from build123d import *
from build123d.topology import SkipClean

# Parameters (mm, degrees)
SKETCH1_R                = 6
BOSS_EXTRUDE1_DEPTH      = 11
SKETCH2_R                = 6
BOSS_EXTRUDE2_DEPTH      = 8
CUT_EXTRUDE1_DEPTH       = 10
CUT_EXTRUDE1_DEPTH_BACK  = 3
SKETCH3_R                = 6
SKETCH3_R_2              = 3
SKETCH5_W                = 8.868099488
SKETCH5_H                = 25.092164851
CUT_EXTRUDE3_DEPTH       = 20.723082923
CUT_EXTRUDE2_START       = -3.3
CUT_EXTRUDE2_DEPTH       = 3.3
CUT_EXTRUDE5_DEPTH       = 2.5
BOSS_EXTRUDE3_REACH      = 18.961
BOSS_EXTRUDE3_END_RADIUS = 6
BOSS_EXTRUDE4_START      = -2.211146
BOSS_EXTRUDE4_DEPTH      = 2.211146
SKETCH10_R               = 3
CUT_EXTRUDE6_DEPTH       = 19.364367672
SKETCH12_R               = 4
SKETCH12_R_2             = 3
BOSS_EXTRUDE5_DEPTH      = 0.3
BOSS_EXTRUDE6_START      = -5
BOSS_EXTRUDE6_DEPTH      = 10
CUT_EXTRUDE12_DEPTH      = 19.364367672
CUT_EXTRUDE9_DEPTH       = 14.244940814
SKETCH15_OUTSIDE_W       = 23.236
SKETCH15_OUTSIDE_H       = 20.984
SKETCH15_OUTSIDE_W_2     = 17.302035992
SKETCH15_OUTSIDE_H_2     = 16.797371099
CUT_EXTRUDE10_DEPTH      = 19.748333259
SKETCH16_R               = 1
CUT_EXTRUDE11_DEPTH      = 19.748333259


with BuildPart() as part:
    # Sketch1 → Boss-Extrude1 (new body)
    with BuildSketch(Plane.XY):
        Circle(SKETCH1_R)
    extrude(amount=BOSS_EXTRUDE1_DEPTH)

    # Sketch2 → Boss-Extrude2 (add, symmetric)
    with BuildSketch(Plane(origin=(0, 0, 0), x_dir=(0, 0, -1), z_dir=(1, 0, 0))):
        Circle(SKETCH2_R)
    extrude(amount=BOSS_EXTRUDE2_DEPTH, both=True)

    # Sketch3 → Cut-Extrude1 (cut, two sides: drawn at the far end of the back side and taken through both)
    with BuildSketch(Plane.ZY.offset(8).offset(-CUT_EXTRUDE1_DEPTH_BACK)):
        with Locations(Location((0, 0, 0), (0, 0, 33.557309762))):
            Circle(SKETCH3_R)
        with Locations(Location((0, 0, 0), (0, 0, 180))):
            Circle(SKETCH3_R_2, mode=Mode.SUBTRACT)
    extrude(amount=CUT_EXTRUDE1_DEPTH + CUT_EXTRUDE1_DEPTH_BACK, mode=Mode.SUBTRACT)

    # Sketch5 → Cut-Extrude3 (cut, through all)
    with BuildSketch(Plane.XY.offset(11)):
        with Locations((4.434049744, 3.885168382)):
            Rectangle(SKETCH5_W, SKETCH5_H)
    extrude(amount=-CUT_EXTRUDE3_DEPTH, mode=Mode.SUBTRACT)

    # Sketch4 → Cut-Extrude2 (cut)
    with BuildSketch(Plane.XY.offset(11).offset(CUT_EXTRUDE2_START)):
        with BuildLine():
            Line((0, 3), (0, 6))
            ThreePointArc((0, 6), (-6, 0), (0, -6))
            Line((0, -6), (0, -3))
            ThreePointArc((0, -3), (-3, 0), (0, 3))
        make_face()
    extrude(amount=CUT_EXTRUDE2_DEPTH, mode=Mode.SUBTRACT)

    # Mirror1: part across plane


with BuildPart() as part_1:
    with SkipClean():  # the faces are left unmerged after this step: merging them gives an invalid solid
        add(part.part)
        add(part.part.mirror(Plane(origin=(0, -8.660914044, -6), x_dir=(0, 0, 1), z_dir=(-1, 0, 0))))

    # Sketch7 → Cut-Extrude5 (cut)
    with BuildSketch(Plane.XY.offset(7.7)):
        with BuildLine():
            Line((-4.535722056, 3.110823914), (-5.732457975, 6))
            Line((-5.732457975, 6), (5.732457975, 6))
            Line((5.732457975, 6), (4.535722056, 3.110823914))
            ThreePointArc((4.535722056, 3.110823914), (0, 5.5), (-4.535722056, 3.110823914))
        make_face()
        with BuildLine():
            Line((4.535722056, -3.110823914), (5.732457975, -6))
            Line((5.732457975, -6), (-5.732457975, -6))
            Line((-5.732457975, -6), (-4.535722056, -3.110823914))
            ThreePointArc((-4.535722056, -3.110823914), (0, -5.5), (4.535722056, -3.110823914))
        make_face()
    extrude(amount=-CUT_EXTRUDE5_DEPTH, mode=Mode.SUBTRACT)

    # Boss-Extrude3: up to this cylinder (the profile starts outside it)
    with SkipClean():  # the faces are left unmerged after this step: merging them gives an invalid solid
        boss_extrude3_end = Plane(origin=(0, 0, 0), z_dir=(1, 0, 0)) * Cylinder(BOSS_EXTRUDE3_END_RADIUS, 63.367438, mode=Mode.PRIVATE)
        # Sketch8 → Boss-Extrude3 (add, up to the surface)
        with BuildSketch(Plane.XY.offset(7.7), mode=Mode.PRIVATE) as boss_extrude3_sk1:
            with BuildLine():
                Line((4.760120042, 3.652568574), (5.402152292, 5.202571539))
                ThreePointArc((5.402152292, 5.202571539), (7.5, 0), (5.402152292, -5.202571539))
                Line((5.402152292, -5.202571539), (4.760120042, -3.652568574))
                ThreePointArc((4.760120042, -3.652568574), (6, 0), (4.760120042, 3.652568574))
            make_face()
        boss_extrude3_tool1 = extrude(boss_extrude3_sk1.sketch, amount=-BOSS_EXTRUDE3_REACH, mode=Mode.PRIVATE) - boss_extrude3_end
        add(boss_extrude3_tool1.solids().sort_by_distance((6.222719, 0, 7.7))[0])
        # Sketch8 → Boss-Extrude3 (add, up to the surface)
        with BuildSketch(Plane.XY.offset(7.7), mode=Mode.PRIVATE) as boss_extrude3_sk2:
            with BuildLine():
                Line((-4.760120042, 3.652568574), (-5.402152292, 5.202571539))
                ThreePointArc((-5.402152292, 5.202571539), (-7.5, 0), (-5.402152292, -5.202571539))
                Line((-5.402152292, -5.202571539), (-4.760120042, -3.652568574))
                ThreePointArc((-4.760120042, -3.652568574), (-6, 0), (-4.760120042, 3.652568574))
            make_face()
        boss_extrude3_tool2 = extrude(boss_extrude3_sk2.sketch, amount=-BOSS_EXTRUDE3_REACH, mode=Mode.PRIVATE) - boss_extrude3_end
        add(boss_extrude3_tool2.solids().sort_by_distance((-6.222719, 0, 7.7))[0])

    # Sketch9 → Boss-Extrude4 (add)
    with SkipClean():  # the faces are left unmerged after this step: merging them gives an invalid solid
        with BuildSketch(Plane.XY.offset(5.2).offset(BOSS_EXTRUDE4_START)):
            with BuildLine():
                Line((2.630513694, 6.350621836), (5.402152292, 5.202571539))
                Line((5.402152292, 5.202571539), (4.760120042, 3.652568574))
                ThreePointArc((4.760120042, 3.652568574), (0, 6), (-4.760120042, 3.652568574))
                Line((-4.760120042, 3.652568574), (-5.402152292, 5.202571539))
                Line((-5.402152292, 5.202571539), (-2.630513694, 6.350621836))
                ThreePointArc((-2.630513694, 6.350621836), (0, 6.873863542), (2.630513694, 6.350621836))
            make_face()
        extrude(amount=BOSS_EXTRUDE4_DEPTH)

    # Sketch10 → Cut-Extrude6 (cut, through all)
    with SkipClean():  # the faces are left unmerged after this step: merging them gives an invalid solid
        with BuildSketch(Plane.ZY.offset(5)):
            with BuildLine():
                ThreePointArc((2.988854192, 5.202571539), (-5.94680377, -0.79719817), (4.25356316, -4.231690023))
                ThreePointArc((4.25356316, -4.231690023), (5.94680377, 0.79719817), (2.988854192, 5.202571539))
            make_face()
            with Locations(Location((0, 0, 0), (0, 0, 180))):
                Circle(SKETCH10_R, mode=Mode.SUBTRACT)
        extrude(amount=CUT_EXTRUDE6_DEPTH, mode=Mode.SUBTRACT)

    # Mirror2: part across plane


with BuildPart() as part_2:
    add(part_1.part)
    add(part_1.part.mirror(Plane.ZX))

    # Sketch12 → Boss-Extrude5 (add)
    with BuildSketch(Plane.XY.offset(7.7)):
        Circle(SKETCH12_R)
        Circle(SKETCH12_R_2, mode=Mode.SUBTRACT)
    extrude(amount=BOSS_EXTRUDE5_DEPTH)

    # Sketch13 → Boss-Extrude6 (add)
    with BuildSketch(Plane(origin=(0, 0, 0), x_dir=(0, 0, -1), z_dir=(1, 0, 0)).offset(BOSS_EXTRUDE6_START)):
        with BuildLine():
            Line((-2.988854192, -6.873863542), (-2.988854192, -5.202571539))
            ThreePointArc((-2.988854192, -5.202571539), (-0.863689726, -5.937511268), (1.38278621, -5.838484589))
            Line((1.38278621, -5.838484589), (-2.988854192, -6.873863542))
        make_face()
        with BuildLine():
            Line((-2.988854192, 5.202571539), (-2.988854192, 6.873863542))
            Line((-2.988854192, 6.873863542), (1.38278621, 5.838484589))
            ThreePointArc((1.38278621, 5.838484589), (-0.863689726, 5.937511268), (-2.988854192, 5.202571539))
        make_face()
    extrude(amount=BOSS_EXTRUDE6_DEPTH)

    # Sketch17 → Cut-Extrude12 (cut, through all)
    with BuildSketch(Plane.ZY.offset(5)):
        with BuildLine():
            Line((2.988854192, -6.873863542), (-2.223044712, -3.912553157))
            ThreePointArc((-2.223044712, -3.912553157), (-4.5, 0), (-2.223044712, 3.912553157))
            Line((-2.223044712, 3.912553157), (2.988854192, 6.873863542))
            Line((2.988854192, 6.873863542), (-1.38278621, 5.838484589))
            ThreePointArc((-1.38278621, 5.838484589), (-6, 0), (-1.38278621, -5.838484589))
            Line((-1.38278621, -5.838484589), (2.988854192, -6.873863542))
        make_face()
    extrude(amount=-CUT_EXTRUDE12_DEPTH, mode=Mode.SUBTRACT)

    # Sketch14 → Cut-Extrude9 (cut, through all)
    with BuildSketch(Plane(origin=(0, 0, 2.988854192), x_dir=(-1, 0, 0), z_dir=(0, 0, -1))):
        with BuildLine():
            Line((5, -16.873863542), (-5, -16.873863542))
            Line((-5, -16.873863542), (-5, -5.369148472))
            Line((-5, -5.369148472), (-2.630513694, -6.350621836))
            ThreePointArc((-2.630513694, -6.350621836), (-1.341024252, -6.741784182), (0, -6.873863542))
            ThreePointArc((0, -6.873863542), (1.341024252, -6.741784182), (2.630513694, -6.350621836))
            Line((2.630513694, -6.350621836), (5, -5.369148472))
            Line((5, -5.369148472), (5, -16.873863542))
        make_face()
    extrude(amount=CUT_EXTRUDE9_DEPTH, mode=Mode.SUBTRACT)

    # Sketch15 outside → Cut-Extrude10 (cut, through all)
    with SkipClean():  # the faces are left unmerged after this step: merging them gives an invalid solid
        with BuildSketch(Plane.XY.offset(11)):
            Rectangle(SKETCH15_OUTSIDE_W, SKETCH15_OUTSIDE_H)
            with Locations((-8.651017996, -8.398685549)):
                Rectangle(SKETCH15_OUTSIDE_W_2, SKETCH15_OUTSIDE_H_2, mode=Mode.SUBTRACT)
        extrude(amount=-CUT_EXTRUDE10_DEPTH, mode=Mode.SUBTRACT)

    # Mirror3: part across plane


with BuildPart() as part_3:
    add(part_2.part)
    add(part_2.part.mirror(Plane(origin=(0, 0, -4.5), x_dir=(0, 0, 1), z_dir=(0, 1, 0))))

    # Mirror4: part across face


with BuildPart() as part_4:
    with SkipClean():  # the faces are left unmerged after this step: merging them gives an invalid solid
        add(part_3.part)
        add(part_3.part.mirror(Plane(origin=(0, 0, 3.307079487), x_dir=(0, 0, 1), z_dir=(1, 0, 0))))

    # Sketch16 → Cut-Extrude11 (cut, through all)
    with SkipClean():  # the faces are left unmerged after this step: merging them gives an invalid solid
        with BuildSketch(Plane.XY.offset(11)):
            Circle(SKETCH16_R)
        extrude(amount=-CUT_EXTRUDE11_DEPTH, mode=Mode.SUBTRACT)


solid = part_4.part
Work out the finished part from the listing and answer in its coordinate system (mm). Round coordinates to 2 decimals unless told otherwise and drop trailing zeros. Order: outer loops, then holes, each group sorted by start corner. A loop starts at its lowest first (then second) coordinate and runs counter-clockwise, first axis right, second up. Notation, with made-up numbers: M 48.5,9.25 L 56.5,9.25 A3 cw 56.5,14.25 Z; hole C 78,-7 d7. An arc over 180 degrees is marked long. One line per item, written item: value.
Q1. Find section B-B on x = 5.75. Write down the section's boundary in (y, z).
Derived:
outline: M -4.82,3.58 A6 cw 4.82,3.58 L 4.82,7.7 L -4.82,7.7 Z; C 0,0 d6
Q2. Find section C-C on z = 1.5. Write down the section's boundary in (x, y), then the cut area to 3 significant figures.
Derived:
outline: M -8,-2.6 L -5,-2.6 L -5,-5.37 L -3.41,-6.03 L 3.41,-6.03 L 5,-5.37 L 5,-2.6 L 8,-2.6 L 8,2.6 L 5,2.6 L 5,5.37 L 3.41,6.03 L -3.41,6.03 L -5,5.37 L -5,2.6 L -8,2.6 Z; hole C 0,0 d2
area: 146 mm²
Q3. Straight lines are drawn through the part: line 1 (Y direction, x = 0, z = 3); line 2 (Y direction, x = 0, z = 6.5); line 3 (X direction, y = 4.5, z = 5.25). For each, find the intervals that lie inside material, in ascending order.
Derived:
line 1: -6.87 to -1, 1 to 6.87
line 2: -5.5 to -1, 1 to 5.5
line 3: -6 to -5.11, -3.16 to 3.16, 5.11 to 6
Q4. Find section A-A on y = -0.25. Write down the section's boundary in (x, z), then the cut area to 3 significant figures.
Derived:
outline: M -8,-2.99 L -5,-2.99 L -5,-4.49 L -0.97,-4.49 L -0.97,11 L -2.99,11 L -2.99,8 L -3.99,8 L -3.99,7.7 L -7.5,7.7 L -7.5,5.99 L -5,5.99 L -5,2.99 L -8,2.99 Z; M 0.97,-4.49 L 5,-4.49 L 5,-2.99 L 8,-2.99 L 8,2.99 L 5,2.99 L 5,5.99 L 7.5,5.99 L 7.5,7.7 L 3.99,7.7 L 3.99,8 L 2.99,8 L 2.99,11 L 0.97,11 Z
area: 157 mm²
Q5. Determine the mould class of faces 1 (the face through (1, 0, 3)), 2 (the face through (0.038, 6.874, 3.96)), 3 (the face through (2, -4, 7.7)) for opening direction X: released by +X, released by -X, zero draft, split by the parting line, or undercut.
Derived:
face 1: undercut
face 2: split by the parting line
face 3: zero draft
Q6. Find section D-D on x = -3.5. Write down the section's boundary in (y, z).
Derived:
outline: M -5.99,1.43 L -3.91,-2.22 A4.5 ccw 3.91,-2.22 L 5.99,1.43 L 5.99,5.2 L 4.24,5.2 L 4.24,7.7 L 1.94,7.7 L 1.94,8 L -1.94,8 L -1.94,7.7 L -4.24,7.7 L -4.24,5.2 L -5.99,5.2 Z
Q7. Flat-ended cylindrical pins translate along their axes: pin 1 (5 mm diameter, centred on x = -6, y = -2.5, fed in from -Z); pin 2 (1.9 mm diameter, centred on x = 1.5, y = 5.5, fed in from +Z); pin 3 (6 mm diameter, centred on x = 1, z = 8.5, fed in from -Y). Find the tip coordinate at first contact, or state that the pin passes through.
Derived:
pin 1: z = -4.5
pin 2: z = 7.7
pin 3: y = -5.5
